Can you work these out from the model? Positions are in its coordinate system, mm. Coordinates: 2 decimals unless noted, no trailing zeros. Order: outer loops, then holes, each group sorted by start corner. A loop starts at its lowest first (then second) coordinate and runs counter-clockwise, first axis right, second up. Notation, with made-up numbers: (-31, 71.5) -> (-22, 71.5) arc R14 ccw to (-22, 82.5) -> close; hole circle Ø10 at (74, -19.75). An arc over 180 degrees is marked (long way). Write item = value, one per line. Start each with the question number.
from build123d import *

# Parameters (mm, degrees)
SKETCH1_R           = 2.1
SKETCH1_R_2         = 1.6
BOSS_EXTRUDE1_DEPTH = 3.175
FILLET1_R           = 3.2


with BuildPart() as part:
    # Sketch1 → Boss-Extrude1 (new body)
    with BuildSketch(Plane(origin=(0, 0, 0), x_dir=(1, 0, 0), z_dir=(0, 1, 0))):
        Polygon((-114, -271), (-70, -271), (-70, 171), (70, 171), (70, -271), (114, -271), (114, 271), (-114, 271), align=None)
        with Locations(Location((106, 261, 0), (0, 0, 270))):
            Circle(SKETCH1_R, mode=Mode.SUBTRACT)
        with Locations(Location((106, 197.5, 0), (0, 0, 270))):
            Circle(SKETCH1_R, mode=Mode.SUBTRACT)
        with Locations(Location((106, 134, 0), (0, 0, 270))):
            Circle(SKETCH1_R, mode=Mode.SUBTRACT)
        with Locations(Location((106, 70.5, 0), (0, 0, 270))):
            Circle(SKETCH1_R, mode=Mode.SUBTRACT)
        with Locations(Location((106, 7, 0), (0, 0, 270))):
            Circle(SKETCH1_R, mode=Mode.SUBTRACT)
        with Locations(Location((106, -56.5, 0), (0, 0, 270))):
            Circle(SKETCH1_R, mode=Mode.SUBTRACT)
        with Locations(Location((106, -120, 0), (0, 0, 270))):
            Circle(SKETCH1_R, mode=Mode.SUBTRACT)
        with Locations(Location((106, -183.5, 0), (0, 0, 270))):
            Circle(SKETCH1_R, mode=Mode.SUBTRACT)
        with Locations(Location((78, -247, 0), (0, 0, 270))):
            Circle(SKETCH1_R, mode=Mode.SUBTRACT)
        with Locations(Location((78, -183.5, 0), (0, 0, 270))):
            Circle(SKETCH1_R, mode=Mode.SUBTRACT)
        with Locations(Location((78, -120, 0), (0, 0, 270))):
            Circle(SKETCH1_R, mode=Mode.SUBTRACT)
        with Locations(Location((78, -56.5, 0), (0, 0, 270))):
            Circle(SKETCH1_R, mode=Mode.SUBTRACT)
        with Locations(Location((78, 7, 0), (0, 0, 270))):
            Circle(SKETCH1_R, mode=Mode.SUBTRACT)
        with Locations(Location((78, 70.5, 0), (0, 0, 270))):
            Circle(SKETCH1_R, mode=Mode.SUBTRACT)
        with Locations(Location((78, 134, 0), (0, 0, 270))):
            Circle(SKETCH1_R, mode=Mode.SUBTRACT)
        with Locations(Location((78, 197.5, 0), (0, 0, 270))):
            Circle(SKETCH1_R, mode=Mode.SUBTRACT)
        with Locations(Location((78, 261, 0), (0, 0, 270))):
            Circle(SKETCH1_R, mode=Mode.SUBTRACT)
        with Locations(Location((92, -29, 0), (0, 0, 270))):
            Circle(SKETCH1_R_2, mode=Mode.SUBTRACT)
        with Locations(Location((92, 206, 0), (0, 0, 270))):
            Circle(SKETCH1_R_2, mode=Mode.SUBTRACT)
        with Locations(Location((92, -264, 0), (0, 0, 270))):
            Circle(SKETCH1_R_2, mode=Mode.SUBTRACT)
        with Locations(Location((-106, 261, 0), (0, 0, 270))):
            Circle(SKETCH1_R, mode=Mode.SUBTRACT)
        with Locations(Location((-78, 261, 0), (0, 0, 270))):
            Circle(SKETCH1_R, mode=Mode.SUBTRACT)
        with Locations(Location((-92, 206, 0), (0, 0, 270))):
            Circle(SKETCH1_R_2, mode=Mode.SUBTRACT)
        with Locations(Location((-78, 70.5, 0), (0, 0, 270))):
            Circle(SKETCH1_R, mode=Mode.SUBTRACT)
        with Locations(Location((-106, 70.5, 0), (0, 0, 270))):
            Circle(SKETCH1_R, mode=Mode.SUBTRACT)
        with Locations(Location((-106, 134, 0), (0, 0, 270))):
            Circle(SKETCH1_R, mode=Mode.SUBTRACT)
        with Locations(Location((-106, 197.5, 0), (0, 0, 270))):
            Circle(SKETCH1_R, mode=Mode.SUBTRACT)
        with Locations(Location((-92, -264, 0), (0, 0, 270))):
            Circle(SKETCH1_R_2, mode=Mode.SUBTRACT)
        with Locations(Location((-92, -29, 0), (0, 0, 270))):
            Circle(SKETCH1_R_2, mode=Mode.SUBTRACT)
        with Locations(Location((-78, 7, 0), (0, 0, 270))):
            Circle(SKETCH1_R, mode=Mode.SUBTRACT)
        with Locations(Location((-78, -56.5, 0), (0, 0, 270))):
            Circle(SKETCH1_R, mode=Mode.SUBTRACT)
        with Locations(Location((-78, -120, 0), (0, 0, 270))):
            Circle(SKETCH1_R, mode=Mode.SUBTRACT)
        with Locations(Location((-78, -183.5, 0), (0, 0, 270))):
            Circle(SKETCH1_R, mode=Mode.SUBTRACT)
        with Locations(Location((-78, -247, 0), (0, 0, 270))):
            Circle(SKETCH1_R, mode=Mode.SUBTRACT)
        with Locations(Location((-106, -247, 0), (0, 0, 270))):
            Circle(SKETCH1_R, mode=Mode.SUBTRACT)
        with Locations(Location((-106, -183.5, 0), (0, 0, 270))):
            Circle(SKETCH1_R, mode=Mode.SUBTRACT)
        with Locations(Location((-106, -120, 0), (0, 0, 270))):
            Circle(SKETCH1_R, mode=Mode.SUBTRACT)
        with Locations(Location((-106, -56.5, 0), (0, 0, 270))):
            Circle(SKETCH1_R, mode=Mode.SUBTRACT)
        with Locations(Location((-106, 7, 0), (0, 0, 270))):
            Circle(SKETCH1_R, mode=Mode.SUBTRACT)
        with Locations(Location((-78, 197.5, 0), (0, 0, 270))):
            Circle(SKETCH1_R, mode=Mode.SUBTRACT)
        with Locations(Location((-78, 134, 0), (0, 0, 270))):
            Circle(SKETCH1_R, mode=Mode.SUBTRACT)
        with Locations(Location((-52, 177, 0), (0, 0, 270))):
            Circle(SKETCH1_R, mode=Mode.SUBTRACT)
        with Locations(Location((-36, 177, 0), (0, 0, 270))):
            Circle(SKETCH1_R, mode=Mode.SUBTRACT)
        with Locations(Location((-36, 231, 0), (0, 0, 270))):
            Circle(SKETCH1_R, mode=Mode.SUBTRACT)
        with Locations(Location((-52, 231, 0), (0, 0, 270))):
            Circle(SKETCH1_R, mode=Mode.SUBTRACT)
        with Locations(Location((36, 177, 0), (0, 0, 270))):
            Circle(SKETCH1_R, mode=Mode.SUBTRACT)
        with Locations(Location((52, 177, 0), (0, 0, 270))):
            Circle(SKETCH1_R, mode=Mode.SUBTRACT)
        with Locations(Location((52, 231, 0), (0, 0, 270))):
            Circle(SKETCH1_R, mode=Mode.SUBTRACT)
        with Locations(Location((36, 231, 0), (0, 0, 270))):
            Circle(SKETCH1_R, mode=Mode.SUBTRACT)
        with Locations(Location((-39, 197.5, 0), (0, 0, 270))):
            Circle(SKETCH1_R, mode=Mode.SUBTRACT)
        with Locations(Location((-39, 261, 0), (0, 0, 270))):
            Circle(SKETCH1_R, mode=Mode.SUBTRACT)
        with Locations(Location((106, -247, 0), (0, 0, 270))):
            Circle(SKETCH1_R, mode=Mode.SUBTRACT)
        with Locations(Location((0, 197.5, 0), (0, 0, 270))):
            Circle(SKETCH1_R, mode=Mode.SUBTRACT)
        with Locations(Location((0, 261, 0), (0, 0, 270))):
            Circle(SKETCH1_R, mode=Mode.SUBTRACT)
        with Locations(Location((39, 197.5, 0), (0, 0, 270))):
            Circle(SKETCH1_R, mode=Mode.SUBTRACT)
        with Locations(Location((39, 261, 0), (0, 0, 270))):
            Circle(SKETCH1_R, mode=Mode.SUBTRACT)
    extrude(amount=BOSS_EXTRUDE1_DEPTH)

    # Fillet1
    fillet1_edges = [part.edges().sort_by_distance(p)[0] for p in [
        (70, 1.5875, -171),
        (-70, 1.5875, -171),
        (-70, 1.5875, 271),
        (-114, 1.5875, 271),
        (-114, 1.5875, -271),
        (114, 1.5875, -271),
        (114, 1.5875, 271),
        (70, 1.5875, 271),
    ]]
    fillet(fillet1_edges, radius=FILLET1_R)


solid = part.part
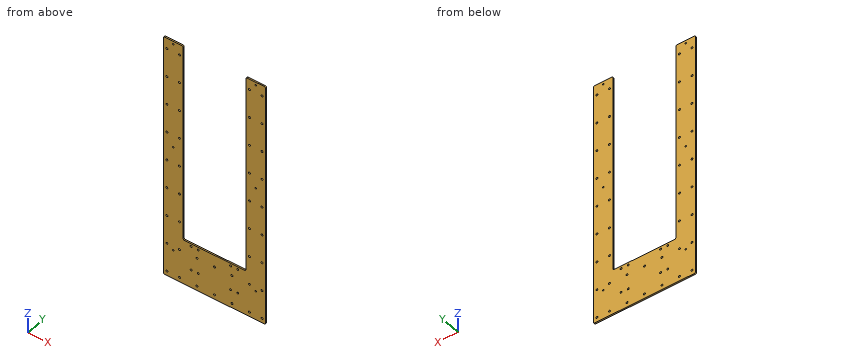
(1) Imagine slicing it at B-B (y = 2.55). Count the separate pieces of the cut face and the enclosed holes in it, plus the area to 3 significant figures.
(2) Imagine slicing it at C-C (x = 13.5). Write out the boundary of the cut face in (y, z) (3 decimals), plus the area to 4 significant figures.
(3) Imagine slicing it at A-A (z = 75.5). Write out the boundary of the cut face in (x, y) (3 decimals), plus the area to 3 significant figures.
(4) If I drill on L1, parallel to X at y = 1.1, z = -70.5; L2, parallel to X at y = 1.5, z = 247.5; L3, parallel to X at y = 2.2, z = -231, over which ranges is the centre line in solid material (lowest first)? Write a range as from..to.
(5) For P1, Ø4, axis at x = 78, z = -261, coming from the -Y side, with a flat end and sliding along its axis, tell me the tip position at first contact or that it passes through.
Result set:
q1.separate_pieces = 1
q1.enclosed_holes = 56
q1.area = 60,900 mm2
q2.outline = (0, -271) -> (3.175, -271) -> (3.175, -171) -> (0, -171) -> close
q2.area = 317.5 mm2
q3.outline = (-114, 0) -> (-70, 0) -> (-70, 3.175) -> (-114, 3.175) -> close; (70, 0) -> (114, 0) -> (114, 3.175) -> (70, 3.175) -> close
q3.area = 279 mm2
q4.L1 = -114..-108.1, -103.9..-80.1, -75.9..-70, 70..75.9, 80.1..103.9, 108.1..114
q4.L2 = -114..-108.04, -103.96..-80.04, -75.96..-70, 70..75.96, 80.04..103.96, 108.04..114
q4.L3 = -114..-54.1, -49.9..-38.1, -33.9..33.9, 38.1..49.9, 54.1..114
q5.P1 = through
